Check sheet for the modelled part. Datum: model origin and axes. Units: mm. Face numbers are marked on the shaded views. A direction names the side the tool comes from. Round coordinates to 2 decimals unless told otherwise and drop trailing zeros. Write each loop counter-clockwise with the first axis right and the second up, starting at its lowest first coordinate (ties: lowest second). Pieces come first, ordered by that corner, then holes.
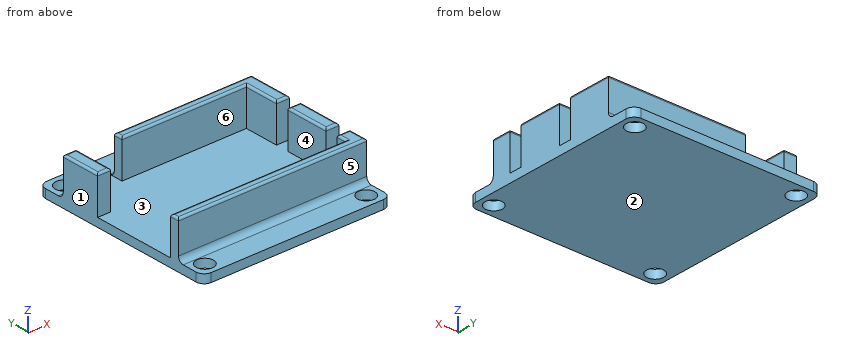
from build123d import *

# Parameters (mm, degrees)
F0_R     = 1.6
F1_DEPTH = 1.6
F2_W     = 2.4
F2_H     = 8.1
F2_H_2   = 1.65
F3_DEPTH = 7
F4_R     = 1
F5_R     = 0.4


with BuildPart() as f1:
    # F0 (on Top) → F1 (new body)
    with BuildSketch(Plane.XY):
        with BuildLine():
            ThreePointArc((-17.5, -16), (-17.0606601718, -17.0606601718), (-16, -17.5))
            Line((-16, -17.5), (16, -17.5))
            ThreePointArc((16, -17.5), (17.0606601718, -17.0606601718), (17.5, -16))
            Line((17.5, -16), (17.5, 16))
            ThreePointArc((17.5, 16), (17.0606601718, 17.0606601718), (16, 17.5))
            Line((16, 17.5), (-16, 17.5))
            ThreePointArc((-16, 17.5), (-17.0606601718, 17.0606601718), (-17.5, 16))
            Line((-17.5, 16), (-17.5, -16))
        make_face()
        with Locations((-15, -15)):
            Circle(F0_R, mode=Mode.SUBTRACT)
        with Locations((15, -15)):
            Circle(F0_R, mode=Mode.SUBTRACT)
        with Locations((-15, 15)):
            Circle(F0_R, mode=Mode.SUBTRACT)
        with Locations((15, 15)):
            Circle(F0_R, mode=Mode.SUBTRACT)
    extrude(amount=F1_DEPTH)

    # F2 (on face) → F3 (join)
    with BuildSketch(Plane.XY.offset(1.6)):
        Polygon((15.1, -10.6), (-15.1, -10.6), (-15.1, -12.25), (17.5, -12.25), (17.5, -8.7), (15.1, -8.7), align=None)
        with Locations((16.3, -2.25)):
            Rectangle(F2_W, F2_H)
        Polygon((-8, 12.25), (-8, 10.6), (15.1, 10.6), (15.1, 4.2), (17.5, 4.2), (17.5, 12.25), align=None)
        Polygon((-17.5, 4.95), (-15.1, 4.95), (-15.1, 10.6), (-15.1, 12.25), (-17.5, 12.25), align=None)
        with Locations((-16.3, -11.425)):
            Rectangle(F2_W, F2_H_2)
    extrude(amount=F3_DEPTH)

    # F4
    f4_edges = [f1.edges().sort_by_distance(p)[0] for p in [
        (0, -12.25, 1.6),
        (4.75, 12.25, 1.6),
        (-16.3, 12.25, 1.6),
    ]]
    fillet(f4_edges, radius=F4_R)

    # F5
    f5_edges = [f1.edges().sort_by_distance(p)[0] for p in [
        (4.75, 12.25, 8.6),
        (3.55, 10.6, 8.6),
        (-15.1, 8.6, 8.6),
        (-17.5, 8.6, 8.6),
        (-16.3, 12.25, 8.6),
        (-8, 11.425, 8.6),
        (-16.3, 4.95, 8.6),
        (-1.2, -10.6, 8.6),
        (0, -12.25, 8.6),
        (16.3, -8.7, 8.6),
        (17.5, -10.475, 8.6),
        (15.1, -9.65, 8.6),
        (16.3, -6.3, 8.6),
        (15.1, -2.25, 8.6),
        (17.5, -2.25, 8.6),
        (16.3, 1.8, 8.6),
        (16.3, 4.2, 8.6),
        (15.1, 7.4, 8.6),
        (17.5, 8.225, 8.6),
        (-17.5, -11.425, 8.6),
    ]]
    fillet(f5_edges, radius=F5_R)


solid = f1.part
1. Sectioned sample at A-A, the plane z = 4. Enter the section's corners in (x, y).
2. Sectioned sample at C-C, the plane y = 6.5. Enter the section's corners in (x, z).
3. Sectioned sample at B-B, the plane y = -15. Enter the section's corners in (x, z), plus the area to 3 significant figures.
4. Go/stop test with flat-tipped pins: pin 1 (4 mm diameter, centred on x = -5, z = 7.5, fed in from -Y); pin 2 (1 mm diameter, centred on x = -3.5, z = 6, fed in from +Y); pin 3 (2 mm diameter, centred on y = -4, z = 6.5, fed in from -X). Record where each tip stops, or that it passes through.
5. Release check for a two-part mould opening along X. For the marked faces 1, 2 and 3 record: released by +X, released by -X, zero draft, split by the parting line, or undercut.
6. Set-up check for the marked faces 4, 5 and 6: record each of +Z, -Z, +X, -X, +Y, -Y from which the full face is reachable in a straight line by a thin tool's end or side.
7. Scan lines: line 1 along Y through (x, z) = (15, 0.85); line 2 along Y through (x, z) = (6, 5.5); line 3 along X through (y, z) = (8.5, 4.5). Record each from-to range of solid material in increasing order.
8. Sectioned sample at D-D, the plane x = -7. Enter the section's corners in (y, z), plus the area to 3 significant figures.
Computed values:
1. outline: (-17.5, -12.25) - (17.5, -12.25) - (17.5, -8.7) - (15.1, -8.7) - (15.1, -10.6) - (-17.5, -10.6) - close; (-17.5, 4.95) - (-15.1, 4.95) - (-15.1, 12.25) - (-17.5, 12.25) - close; (-8, 10.6) - (15.1, 10.6) - (15.1, 4.2) - (17.5, 4.2) - (17.5, 12.25) - (-8, 12.25) - close; (15.1, -6.3) - (17.5, -6.3) - (17.5, 1.8) - (15.1, 1.8) - close
2. outline: (-17.5, 0) - (17.5, 0) - (17.5, 8.2) arc R0.4 ccw to (17.1, 8.6) - (15.5, 8.6) arc R0.4 ccw to (15.1, 8.2) - (15.1, 1.6) - (-15.1, 1.6) - (-15.1, 8.2) arc R0.4 ccw to (-15.5, 8.6) - (-17.1, 8.6) arc R0.4 ccw to (-17.5, 8.2) - close
3. outline: (-17.5, 0) - (-16.6, 0) - (-16.6, 1.6) - (-17.5, 1.6) - close; (-13.4, 0) - (13.4, 0) - (13.4, 1.6) - (-13.4, 1.6) - close; (16.6, 0) - (17.5, 0) - (17.5, 1.6) - (16.6, 1.6) - close
3. area: 45.8 mm2
4. pin 1: stops at y = -12.25
4. pin 2: stops at y = 12.25
4. pin 3: stops at x = 15.1
5. face 1: released by -X
5. face 2: zero draft
5. face 3: undercut
6. face 4: +Z, -X
6. face 5: +Z, +X, -X, -Y
6. face 6: +Z
7. line 1: y = -17.5 to -16.6, -13.4 to 13.4, 16.6 to 17.5
7. line 2: y = -12.25 to -10.6, 10.6 to 12.25
7. line 3: x = -17.5 to -15.1, 15.1 to 17.5
8. outline: (-17.5, 0) - (17.5, 0) - (17.5, 1.6) - (13.25, 1.6) arc R1 cw to (12.25, 2.6) - (12.25, 8.2) arc R0.4 ccw to (11.85, 8.6) - (11, 8.6) arc R0.4 ccw to (10.6, 8.2) - (10.6, 1.6) - (-10.6, 1.6) - (-10.6, 8.2) arc R0.4 ccw to (-11, 8.6) - (-11.85, 8.6) arc R0.4 ccw to (-12.25, 8.2) - (-12.25, 2.6) arc R1 cw to (-13.25, 1.6) - (-17.5, 1.6) - close
8. area: 79.4 mm2
